Read the model definition and answer for the solid it produces. Units are mm, in the model's axes. A direction names the side the tool comes from. Coordinates: 2 decimals unless noted, no trailing zeros. Write each loop counter-clockwise with the first axis right and the second up, starting at its lowest first coordinate (ties: lowest second). Pieces come first, ordered by that corner, then holes. Notation, with made-up numbers: (-18, -8) -> (30, -8) arc R20 ccw to (30, 20) -> close; hole circle Ø11 at (-36, 71.25). An arc over 180 degrees is marked (long way). Return JSON: item names as keys, results as strings.
from build123d import *

# Parameters (mm, degrees)
F0_W     = 99
F0_H     = 6
F1_DEPTH = 48
F3_DEPTH = 15.5
F4_W     = 2
F4_H     = 42
F4_W_2   = 87
F5_DEPTH = 17.5
F6_DEPTH = 6
F7_R     = 2.99999


# Not quite as in the source:
# - a fillet or chamfer is up to 0.001 mm smaller than in the source, because OpenCascade refuses the exact size


with BuildPart() as f1:
    # F0 (on Front) → F1 (new body)
    with BuildSketch(Plane.XZ):
        with Locations((0, 3)):
            Rectangle(F0_W, F0_H)
    extrude(amount=F1_DEPTH)

    # F2 (on face) → F3 (join)
    with BuildSketch(Plane.XY.offset(6)):
        Polygon((49.5, -3), (49.5, 0), (43.5, 0), (-43.5, 0), (-49.5, 0), (-49.5, -3), (-49.5, -48), (-43.5, -48), (-43.5, -3), (43.5, -3), (43.5, -48), (49.5, -48), align=None)
    extrude(amount=F3_DEPTH)

    # F4 (on face) → F5 (cut)
    with BuildSketch(Plane.XY.offset(21.5)):
        with Locations((-44.5, -24)):
            Rectangle(F4_W, F4_H)
        with Locations((0, -24)):
            Rectangle(F4_W_2, F4_H)
        with Locations((44.5, -24)):
            Rectangle(F4_W, F4_H)
    extrude(amount=-F5_DEPTH, mode=Mode.SUBTRACT)

    # F4 (on face) → F6 (join)
    with BuildSketch(Plane.XY.offset(21.5)):
        Polygon((-49.5, -3), (-45.5, -3), (-43.5, -3), (43.5, -3), (45.5, -3), (49.5, -3), (49.5, 0), (-49.5, 0), align=None)
    extrude(amount=F6_DEPTH)

    # F7 (radius 3 in the source; OpenCascade refuses exactly that, so slightly less here)
    f7_edges = [f1.edges().sort_by_distance(p)[0] for p in [
        (-49.5, -48, 10.75),
        (49.5, -48, 10.75),
        (49.5, 0, 13.75),
        (-49.5, 0, 13.75),
    ]]
    fillet(f7_edges, radius=F7_R)


solid = f1.part
1. The part is cut by section C-C (y = -5.5). Determine the outline of the cut face in (x, z), then the cut area to 3 significant figures.
Taken from the geometry:
{"outline": "(-49.5, 0) -> (49.5, 0) -> (49.5, 21.5) -> (45.5, 21.5) -> (45.5, 4) -> (-45.5, 4) -> (-45.5, 21.5) -> (-49.5, 21.5) -> close", "area": "536 mm2"}
2. A tool of negligible diameter and unlimited length cuts with its end or side. For faces 1 (the face through (-47, -25, 21.5)), 2 (the face through (-1, -46, 6)), 3 (the face through (45.5, -24, 13)), from which of +Z, -Z, +X, -X, +Y, -Y can it reach the whole face along a straight path? Write none if from no direction.
Taken from the geometry:
{"face 1": "+Z, +X, -X, -Y", "face 2": "+Z, -Y", "face 3": "+Z"}
3. The part is cut by section B-B (x = -29.5). Determine the outline of the cut face in (y, z).
Taken from the geometry:
{"outline": "(-48, 0) -> (0, 0) -> (0, 27.5) -> (-3, 27.5) -> (-3, 4) -> (-45, 4) -> (-45, 6) -> (-48, 6) -> close"}
4. Consider L1, parallel to X at y = -31.5, z = 19.5; L2, parallel to Y at x = -44, z = 15.5; L3, parallel to Z at x = 20.5, y = -7. Determine where each line is inside the solid, lowest interval first.
Taken from the geometry:
{"L1": "x = -49.5 to -45.5, 45.5 to 49.5", "L2": "y = -48 to -45, -3 to 0", "L3": "z = 0 to 4"}
5. The part is cut by section A-A (z = 20.25). Determine the outline of the cut face in (x, y).
Taken from the geometry:
{"outline": "(-49.5, -45) arc R3 ccw to (-46.5, -48) -> (-43.5, -48) -> (-43.5, -45) -> (-45.5, -45) -> (-45.5, -3) -> (45.5, -3) -> (45.5, -45) -> (43.5, -45) -> (43.5, -48) -> (46.5, -48) arc R3 ccw to (49.5, -45) -> (49.5, -3) arc R3 ccw to (46.5, 0) -> (-46.5, 0) arc R3 ccw to (-49.5, -3) -> close"}
6. Flat-ended cylindrical pins translate along their axes: pin 1 Ø3 at (x, z) = (-17, 12.5) entering from -Y; pin 2 Ø1.5 at (y, z) = (-46.5, 15.5) entering from -X; pin 3 Ø1.8 at (x, y) = (-47.5, -20) entering from +Z. Find the tip coordinate at first contact, or state that the pin passes through.
Taken from the geometry:
{"pin 1": "stops at y = -3", "pin 2": "stops at x = -49.4", "pin 3": "stops at z = 21.5"}
7. For a pull along X with two mould halves and no side action, classify faces 4 (the face through (-1, -1, 27.5)), 5 (the face through (48.6, -0.86, 13.94)), 6 (the face through (-1, -3, 16)) as +X half, -X half, draft (parallel to the pull), parting line (faces both ways), or undercut.
Taken from the geometry:
{"face 4": "draft", "face 5": "+X half", "face 6": "undercut"}
